The listing builds one solid part. Answer for the finished solid, in the listing's coordinates (mm). A direction names the side the tool comes from. Give positions to 0.01 mm unless a question says otherwise; leave off trailing zeros. Write each loop counter-clockwise with the first axis right and the second up, starting at its lowest first coordinate (ties: lowest second). Pieces come first, ordered by that corner, then holes. Notation, with made-up numbers: (-3.75, -7) -> (31.25, -7) arc R35 cw to (31.25, 31) -> close; hole circle Ø10 at (-23.5, -27.5). An arc over 180 degrees is marked (long way). Use CSV: the item, a comma, the result in double quotes. Start each with the question number.
from build123d import *

# Parameters (mm, degrees)
SKETCH1_R                = 2.5
SKETCH1_R_2              = 1.5
BOSS_EXTRUDE2_DEPTH      = 1.95
SKETCH7_W                = 5
SKETCH7_H                = 10
BOSS_EXTRUDE3_DEPTH      = 1
BOSS_EXTRUDE3_DEPTH_BACK = 1
SKETCH8_W                = 1.95
SKETCH8_H                = 2
BOSS_EXTRUDE4_DEPTH      = 0.208712
SKETCH10_R               = 2.5
SKETCH10_R_2             = 1.5
BOSS_EXTRUDE5_DEPTH      = 1.95
SKETCH12_R               = 2.5
SKETCH12_R_2             = 1.5
BOSS_EXTRUDE6_DEPTH      = 0.975
BOSS_EXTRUDE6_DEPTH_BACK = 0.975
SKETCH13_W               = 1.95
SKETCH13_H               = 2.002875352
SKETCH13_H_2             = 2
BOSS_EXTRUDE7_DEPTH      = 0.209969
SKETCH15_R               = 1.5
BOSS_EXTRUDE8_DEPTH      = 0.2
SKETCH16_R               = 1
CUT_EXTRUDE1_DEPTH       = 10
SKETCH17_W               = 5
SKETCH17_H               = 5.480011174
CUT_EXTRUDE2_DEPTH       = 0.1
SKETCH18_W               = 5
SKETCH18_H               = 5.210920168
CUT_EXTRUDE3_DEPTH       = 0.1
SKETCH19_W               = 5
SKETCH19_H               = 5
CUT_EXTRUDE5_DEPTH       = 0.1
SKETCH20_W               = 5
SKETCH20_H               = 5.52517398
CUT_EXTRUDE6_DEPTH       = 0.1


with BuildPart() as part:
    # Sketch1 → Boss-Extrude2 (new body)
    with BuildSketch(Plane.XY):
        Circle(SKETCH1_R)
        Circle(SKETCH1_R_2, mode=Mode.SUBTRACT)
    extrude(amount=BOSS_EXTRUDE2_DEPTH)



with BuildPart() as body_2:
    # Sketch7 → Boss-Extrude3 (new body, two sides)
    with BuildSketch(Plane(origin=(0, 0, 0), x_dir=(1, 0, 0), z_dir=(0, 1, 0))) as boss_extrude3_sk:
        with Locations((-5, -5)):
            Rectangle(SKETCH7_W, SKETCH7_H)
    extrude(amount=BOSS_EXTRUDE3_DEPTH)
    extrude(boss_extrude3_sk.sketch, amount=-BOSS_EXTRUDE3_DEPTH_BACK)


with BuildPart() as part_1:
    add(part.part)

    add(body_2.part)  # Boss-Extrude4 merges body 2
    # Sketch8 → Boss-Extrude4 (add)
    with BuildSketch(Plane(origin=(-2.5, 0, 0), x_dir=(0, 0, -1), z_dir=(1, 0, 0))):
        with Locations((-0.975, 0)):
            Rectangle(SKETCH8_W, SKETCH8_H)
    extrude(amount=BOSS_EXTRUDE4_DEPTH)



with BuildPart() as body_2_2:
    # Sketch10 → Boss-Extrude5 (new body)
    with BuildSketch(Plane.XY.offset(10)):
        Circle(SKETCH10_R)
        Circle(SKETCH10_R_2, mode=Mode.SUBTRACT)
    extrude(amount=-BOSS_EXTRUDE5_DEPTH)


with BuildPart() as body_3:
    # Sketch12 → Boss-Extrude6 (new body, two sides)
    with BuildSketch(Plane.YX.offset(-5)) as boss_extrude6_sk:
        Circle(SKETCH12_R)
        Circle(SKETCH12_R_2, mode=Mode.SUBTRACT)
    extrude(amount=BOSS_EXTRUDE6_DEPTH)
    extrude(boss_extrude6_sk.sketch, amount=-BOSS_EXTRUDE6_DEPTH_BACK)


with BuildPart() as part_2:
    add(part_1.part)

    add(body_2_2.part)  # Boss-Extrude7 merges body 2 2

    add(body_3.part)  # Boss-Extrude7 merges body 3
    # Sketch13 → Boss-Extrude7 (add)
    with BuildSketch(Plane(origin=(-2.5, 0, 0), x_dir=(0, 0, -1), z_dir=(1, 0, 0))):
        with Locations((-5, 0.001437676)):
            Rectangle(SKETCH13_W, SKETCH13_H)
        with Locations((-9.025, 0)):
            Rectangle(SKETCH13_W, SKETCH13_H_2)
    extrude(amount=BOSS_EXTRUDE7_DEPTH)

    # Sketch15 → Boss-Extrude8 (add)
    with BuildSketch(Plane(origin=(0, 0, 0), x_dir=(-1, 0, 0), z_dir=(0, 0, -1))):
        Circle(SKETCH15_R)
    extrude(amount=-BOSS_EXTRUDE8_DEPTH)

    # Sketch16 → Cut-Extrude1 (cut)
    with BuildSketch(Plane(origin=(0, 1, 0), x_dir=(1, 0, 0), z_dir=(0, 1, 0))):
        with Locations((-4.895643924, -7.484223199)):
            Circle(SKETCH16_R)
        with Locations((-4.895643924, -2.515776801)):
            Circle(SKETCH16_R)
    extrude(amount=-CUT_EXTRUDE1_DEPTH, mode=Mode.SUBTRACT)

    # Sketch17 → Cut-Extrude2 (cut)
    with BuildSketch(Plane(origin=(0, 0, 8.05), x_dir=(-1, 0, 0), z_dir=(0, 0, -1))):
        Rectangle(SKETCH17_W, SKETCH17_H)
    extrude(amount=-CUT_EXTRUDE2_DEPTH, mode=Mode.SUBTRACT)

    # Sketch18 → Cut-Extrude3 (cut)
    with BuildSketch(Plane.XY.offset(5.975)):
        Rectangle(SKETCH18_W, SKETCH18_H)
    extrude(amount=-CUT_EXTRUDE3_DEPTH, mode=Mode.SUBTRACT)

    # Sketch19 → Cut-Extrude5 (cut)
    with BuildSketch(Plane(origin=(0, 0, 4.025), x_dir=(-1, 0, 0), z_dir=(0, 0, -1))):
        Rectangle(SKETCH19_W, SKETCH19_H)
    extrude(amount=-CUT_EXTRUDE5_DEPTH, mode=Mode.SUBTRACT)

    # Sketch20 → Cut-Extrude6 (cut)
    with BuildSketch(Plane.XY.offset(1.95)):
        Rectangle(SKETCH20_W, SKETCH20_H)
    extrude(amount=-CUT_EXTRUDE6_DEPTH, mode=Mode.SUBTRACT)


solid = part_2.part
Q1. Section A-A on x = 0 is taken. Give the vertices of the cut face in (y, z) (3 decimals), then the cut area to 3 significant figures.
Q2. Straight lines are drawn through the part: L1, parallel to Z at x = -2, y = 0.4 (3 decimals); L2, parallel to X at y = 0, z = 1; L3, parallel to Z at x = -5, y = 0.5. For each, find the intervals that lie inside material, in ascending order.
Q3. For faces 4 (the face through (-1.5, 0.07, 1.01)), 5 (the face through (-5, -1, 5)), 6 (the face through (2, 0, 1.85)), determine the directions among +Z, -Z, +X, -X, +Y, -Y from which every point of the face is accessible in a straight line to the end or side of a thin tool.
Q4. Section B-B on y = 0 is taken. Give the vertices of the cut face in (x, z) (3 decimals).
Q5. The mould has two halves that part along X. Classify faces 1 (the face through (2.5, -0.1, 0.9)), 2 (the face through (-5, 1, 5)), 3 (the face through (-3.942, 0.014, 7.184)): +X half, -X half, draft (parallel to the pull), parting line (faces both ways), or undercut.
Q6. Section D-D on x = -2 is taken. Give the vertices of the cut face in (y, z) (3 decimals).
Q7. Flat-ended cylindrical pins translate along their axes: pin 1 Ø1.5 at (x, z) = (-2, 6) entering from +Y; pin 2 Ø1.6 at (x, z) = (-4.9, 7.48) entering from -Y; pin 3 Ø0.6 at (y, z) = (0, 7) entering from +X; pin 4 Ø5 at (x, z) = (-5, 8) entering from +Y. Find the tip coordinate at first contact, or state that the pin passes through.
Output:
1,outline,"(-2.5, 0) -> (2.5, 0) -> (2.5, 1.85) -> (1.5, 1.85) -> (1.5, 0.2) -> (-1.5, 0.2) -> (-1.5, 1.85) -> (-2.5, 1.85) -> close; (-2.5, 4.125) -> (-1.5, 4.125) -> (-1.5, 5.875) -> (-2.5, 5.875) -> close; (-2.5, 8.15) -> (-1.5, 8.15) -> (-1.5, 10) -> (-2.5, 10) -> close; (1.5, 4.125) -> (2.5, 4.125) -> (2.5, 5.875) -> (1.5, 5.875) -> close; (1.5, 8.15) -> (2.5, 8.15) -> (2.5, 10) -> (1.5, 10) -> close"
1,area,"11.5 mm²"
2,L1,"0 to 1.85, 4.125 to 5.875, 8.15 to 10"
2,L2,"-7.5 to -1.5, 1.5 to 2.5"
2,L3,"0 to 1.52, 3.51 to 6.49, 8.48 to 10"
3,face 4,"+Z"
3,face 5,"+Z, -Z, -X, -Y"
3,face 6,"+X, +Y, -Y"
4,outline,"(-7.5, 0) -> (2.5, 0) -> (2.5, 1.85) -> (1.5, 1.85) -> (1.5, 0.2) -> (-1.5, 0.2) -> (-1.5, 1.85) -> (-2.5, 1.85) -> (-2.5, 4.125) -> (-1.5, 4.125) -> (-1.5, 5.875) -> (-2.5, 5.875) -> (-2.5, 8.15) -> (-1.5, 8.15) -> (-1.5, 10) -> (-7.5, 10) -> close; (1.5, 4.125) -> (2.5, 4.125) -> (2.5, 5.875) -> (1.5, 5.875) -> close; (1.5, 8.15) -> (2.5, 8.15) -> (2.5, 10) -> (1.5, 10) -> close; hole circle Ø2 at (-4.896, 2.516); hole circle Ø2 at (-4.896, 7.484)"
5,face 1,"parting line"
5,face 2,"draft"
5,face 3,"undercut"
6,outline,"(-1.5, 0) -> (1.5, 0) -> (1.5, 1.85) -> (-1.5, 1.85) -> close; (-1.5, 4.125) -> (1.5, 4.125) -> (1.5, 5.875) -> (-1.5, 5.875) -> close; (-1.5, 8.15) -> (1.5, 8.15) -> (1.5, 10) -> (-1.5, 10) -> close"
7,pin 1,"y = 2.16"
7,pin 2,"through"
7,pin 3,"x = -2.5"
7,pin 4,"y = 1"
